Job drawing, mm, ordinate dimensions from the low corner. One solid piece. Give positions to 0.01 mm unless a question says otherwise; leave off trailing zeros. Order: outer loops, then holes, each group sorted by start corner. A loop starts at its lowest first (then second) coordinate and runs counter-clockwise, first axis right, second up.
1. Slice it at D-D on z = 4.5. List the corners of the cut face in (x, y).
2. Slice it at A-A on y = 20. List the corners of the cut face in (x, z), and give its area (3 significant figures).
3. Probe line 1 (X direction, y = 20.5, z = 7.25); line 2 (Y direction, x = 77.5, z = 4); line 3 (X direction, y = 25, z = 12) (1 decimal). List the from-to ranges inside material, lowest first.
4. Slice it at C-C on z = 10.75. List the corners of the cut face in (x, y).
5. Drop flat-ended pins along their axis: pin 1 Ø17.5 at (x, y) = (74, 19) entering from -Z; pin 2 Ø19.5 at (x, y) = (77.5, 20) entering from -Z. Give the stop position or say it passes through.
6. Slice it at B-B on x = 77.5. List the corners of the cut face in (y, z).
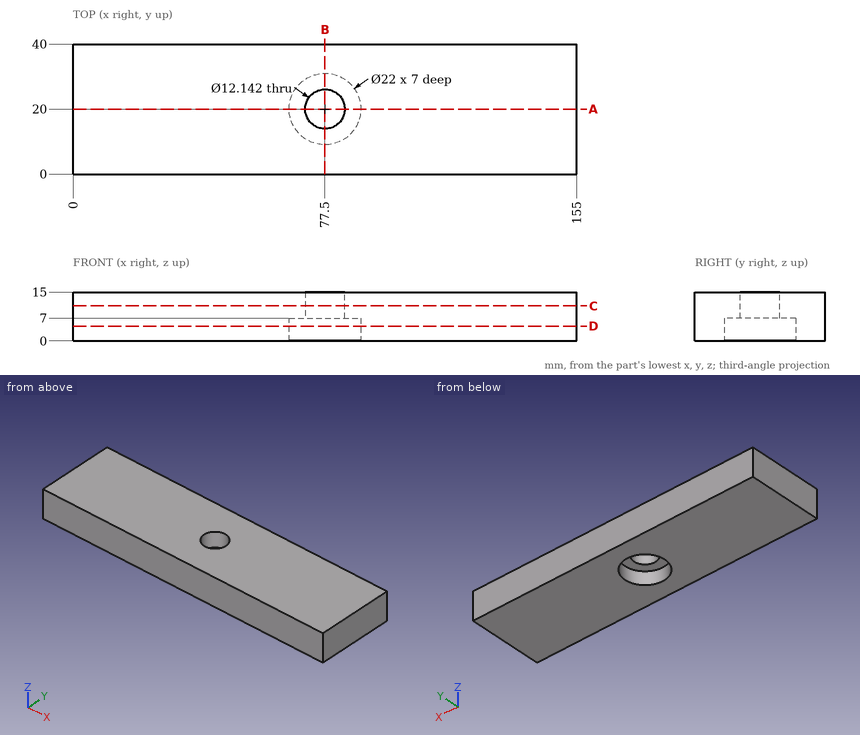
Data:
1. outline: (0, 0) - (155, 0) - (155, 40) - (0, 40) - close; hole circle Ø22 at (77.5, 20)
2. outline: (0, 0) - (66.5, 0) - (66.5, 7) - (71.43, 7) - (71.43, 15) - (0, 15) - close; (83.57, 7) - (88.5, 7) - (88.5, 0) - (155, 0) - (155, 15) - (83.57, 15) - close
2. area: 2,070 mm2
3. line 1: x = 0 to 71.45, 83.55 to 155
3. line 2: y = 0 to 9, 31 to 40
3. line 3: x = 0 to 74.1, 80.9 to 155
4. outline: (0, 0) - (155, 0) - (155, 40) - (0, 40) - close; hole circle Ø12.14 at (77.5, 20)
5. pin 1: stops at z = 0
5. pin 2: stops at z = 7
6. outline: (0, 0) - (9, 0) - (9, 7) - (13.93, 7) - (13.93, 15) - (0, 15) - close; (26.07, 7) - (31, 7) - (31, 0) - (40, 0) - (40, 15) - (26.07, 15) - close
